from build123d import *

# Parameters (mm, degrees)
BOSS_EXTRU_1_DEPTH      = 5
ESQUISSE2_W             = 30
ESQUISSE2_H             = 30
ESQUISSE2_W_2           = 20
ESQUISSE2_H_2           = 20
BOSS_EXTRU_2_DEPTH      = 1
ESQUISSE3_W             = 5
ESQUISSE3_H             = 5.2
ESQUISSE3_W_2           = 5.2
ESQUISSE3_H_2           = 5
ENL_V_MAT_EXTRU_1_DEPTH = 4.8
CONG_1_R                = 1
CONG_2_R                = 0.5


with BuildPart() as part:
    # Esquisse1 → Boss.-Extru.1 (new body)
    with BuildSketch(Plane(origin=(0, 0, 0), x_dir=(1, 0, 0), z_dir=(0, 1, 0))):
        Polygon((22, 13), (12.003020456, 23), (-12.003020456, 23), (-22, 13), (-22, -13), (-12.003020456, -23), (12.003020456, -23), (22, -13), (22, -5), (26, -5), (26, 5), (22, 5), align=None)
    extrude(amount=BOSS_EXTRU_1_DEPTH)

    # Esquisse2 → Boss.-Extru.2 (add)
    with BuildSketch(Plane(origin=(0, 5, 0), x_dir=(1, 0, 0), z_dir=(0, 1, 0))):
        with Locations((1.645517895, 0)):
            Rectangle(ESQUISSE2_W, ESQUISSE2_H)
        with Locations((1.645517895, 0)):
            Rectangle(ESQUISSE2_W_2, ESQUISSE2_H_2, mode=Mode.SUBTRACT)
    extrude(amount=BOSS_EXTRU_2_DEPTH)

    # Esquisse3 → Enlèv. mat.-Extru.1 (cut)
    with BuildSketch(Plane.XZ):
        with Locations((-13.5, 14.4)):
            Rectangle(ESQUISSE3_W, ESQUISSE3_H)
        with Locations((-13.4, -14.4)):
            Rectangle(ESQUISSE3_W_2, ESQUISSE3_H)
        with Locations((14.4, -14.4)):
            Rectangle(ESQUISSE3_W_2, ESQUISSE3_H)
        with Locations((13.4, 14.4)):
            Rectangle(ESQUISSE3_W_2, ESQUISSE3_H)
        Rectangle(ESQUISSE3_W, ESQUISSE3_H_2)
    extrude(amount=-ENL_V_MAT_EXTRU_1_DEPTH, mode=Mode.SUBTRACT)

    # Congé1
    cong_1_edges = [part.edges().sort_by_distance(p)[0] for p in [
        (16.645517895, 5.5, -15),
        (-13.354482105, 5.5, -15),
        (-13.354482105, 5.5, 15),
        (16.645517895, 5.5, 15),
    ]]
    fillet(cong_1_edges, radius=CONG_1_R)

    # Congé2
    cong_2_edges = [part.edges().sort_by_distance(p)[0] for p in [
        (-8.354482105, 5.5, -10),
        (-8.354482105, 5.5, 10),
        (11.645517895, 5.5, 10),
        (11.645517895, 5.5, -10),
    ]]
    fillet(cong_2_edges, radius=CONG_2_R)


solid = part.part
Geometry: final body of the model. Coordinates: model frame, mm. A direction names the side the tool comes from. Give positions to 0.01 mm unless a question says otherwise; leave off trailing zeros. Order: outer loops, then holes, each group sorted by start corner. A loop starts at its lowest first (then second) coordinate and runs counter-clockwise, first axis right, second up. Notation, with made-up numbers: (-29, -16) -> (3, -16) arc R10 cw to (3, -12) -> close; hole circle Ø3 at (-26.75, 67.25). An arc over 180 degrees is marked (long way). Write each question's results on one line, items separated by ' | '.
1) Cut plane A-A (z = -0.5). Output: boundary loops of the cut face in (x, y).
Geometry says:
outline: (-22, 0) -> (-2.5, 0) -> (-2.5, 4.8) -> (2.5, 4.8) -> (2.5, 0) -> (26, 0) -> (26, 5) -> (16.65, 5) -> (16.65, 6) -> (11.65, 6) -> (11.65, 5) -> (-8.35, 5) -> (-8.35, 6) -> (-13.35, 6) -> (-13.35, 5) -> (-22, 5) -> close
2) Set-up query: faces 4 (the face through (24, 2, -5)), 5 (the face through (-22, 2, 0)), 6 (the face through (-2.5, 2, 0)), 7 (the face through (24, 2, 5)), 8 (the face through (26, 2, 0)). Return all of +Z, -Z, +X, -X, +Y, -Y with unobstructed straight access to the full face (end or side cutting, diameter ignored); none if empty.
Geometry says:
face 4: -Z, +X, +Y, -Y | face 5: +Z, -Z, -X, +Y, -Y | face 6: -Y | face 7: +Z, +X, +Y, -Y | face 8: +Z, -Z, +X, +Y, -Y
3) Cut plane D-D (z = 8). Output: boundary loops of the cut face in (x, y), and give its area (3 significant figures).
Geometry says:
outline: (-22, 0) -> (22, 0) -> (22, 5) -> (16.65, 5) -> (16.65, 6) -> (11.65, 6) -> (11.65, 5) -> (-8.35, 5) -> (-8.35, 6) -> (-13.35, 6) -> (-13.35, 5) -> (-22, 5) -> close | area: 230 mm²
4) Cut plane B-B (y = 1.15). Give the number of separate pieces and of enclosed holes in the cut face, and give its area (3 significant figures).
Geometry says:
separate pieces: 1 | enclosed holes: 5 | area: 1,730 mm²
5) Draft query along X for faces 1 (the face through (17, 2, -18)), 2 (the face through (0, 2, -2.5)), 3 (the face through (-17, 2, -18)). Return one class per face: released by +X, released by -X, zero draft, split by the parting line, or undercut.
Geometry says:
face 1: released by +X | face 2: undercut | face 3: released by -X
6) Line query: line 1 along X through (y, z) = (4.7, -12.5); line 2 along X through (y, z) = (3.55, 12.5); line 3 along X through (y, z) = (0.5, -1). Output: solid intervals per line, ascending.
Geometry says:
line 1: x = -22 to -16, -10.8 to 11.8, 17 to 22 | line 2: x = -22 to -16, -11 to 10.8, 16 to 22 | line 3: x = -22 to -2.5, 2.5 to 26
7) Cut plane C-C (x = -10). Output: boundary loops of the cut face in (y, z).
Geometry says:
outline: (0, -23) -> (5, -23) -> (5, -15) -> (6, -15) -> (6, 15) -> (5, 15) -> (5, 23) -> (0, 23) -> close
8) First-contact query: pin 1 Ø1.5 at (x, z) = (-16, 8) entering from +Y; pin 2 Ø2.5 at (x, z) = (14, -13.5) entering from -Y; pin 3 Ø2 at (y, z) = (4.5, -11.5) entering from +X. Flat tips, straight axial feed; report the tip coordinate or a pass-through.
Geometry says:
pin 1: stops at y = 5 | pin 2: stops at y = 4.8 | pin 3: stops at x = 22
